Autodesk Inventor part; units mm, degrees
ref_plane "YZ Plane" through (0, 0, 0) normal (1, 0, 0) x (0, 1, 0)
ref_plane "XZ Plane" through (0, 0, 0) normal (0, 1, 0) x (-1, 0, 0)
ref_plane "XY Plane" through (0, 0, 0) normal (0, 0, 1) x (1, 0, 0)
sketch "Szkic2" plane through (0, 0, 0) normal (1, 0, 0) x (0, 1, 0)
  line L0 (0, -2.9) -> (0, 2.9)
  line L1 (-1.5, -1.5) -> (-1.5, 1.5)
  line L2 (-1.5, -1.5) -> (0, -2.9)
  line L3 (-1.5, 1.5) -> (0, 2.9)
  line L4 (0, 0) -> (-6, 0)
  line L5 (-6, 0) -> (-6, -1.5)
  line L6 (-6, -1.5) -> (-1.5, -1.5)
  dimension "d0" = 5.8
  dimension "d2" = 3
  dimension "d3" = 1.5
  dimension "d4" = 6
  dimension "d5" = 1.5
revolve "Obrót1" add sketch "Szkic2" angle 360 about axis through (0, 0, 0) along (0, -1, 0) contours L2 L1 L4 L0 | L6 L5 L4 L1
sketch "Szkic3" plane through (0, 0, 0) normal (0, 1, 0) x (1, 0, 0)
  line L0 (-1.1673, -0.633) -> (-1.1318, 0.6945)
  line L1 (-1.1318, 0.6945) -> (0.0355, 1.3274)
  line L2 (0.0355, 1.3274) -> (1.1673, 0.633)
  line L3 (1.1673, 0.633) -> (1.1318, -0.6945)
  line L4 (1.1318, -0.6945) -> (-0.0355, -1.3274)
  line L5 (-0.0355, -1.3274) -> (-1.1673, -0.633)
  point P0 (0, 0)
  point P1 (0, 0)
  dimension "d7" = 2.3
extrude "Wyciągnięcie proste1" cut sketch "Szkic3" against normal blind 2
fillet "Zaokrąglenie1" radius 0.5 6 edges at (-1.1496, -2, -0.0308) (-0.6014, -2, 0.9802) (-0.5482, -2, -1.011) (0.6014, -2, -0.9802) (0.5482, -2, 1.011) (1.1496, -2, 0.0308)
fillet "Zaokrąglenie2" radius 0.5 1 edges at (0, -1.5, 1.5)
fillet "Zaokrąglenie3" radius 0.1 1 edges at (0, 0, 2.9)
thread "Gwint1"
chamfer "Faza1" distance 0.5 angle 45 1 edges at (0, -6, 1.5)
properties part number "Screw M3 6mm flat head"
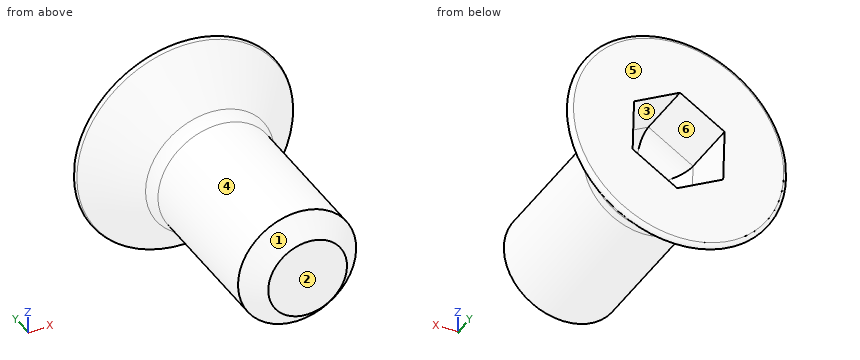
The listing builds one solid part. Answer for the finished solid, in the listing's coordinates (mm). Face numbers are marked on the shaded views. A direction names the side the tool comes from. Round coordinates to 2 decimals unless told otherwise and drop trailing zeros. Loops run counter-clockwise (first coordinate to the right, second up) from the corner with the lowest first, then second, coordinate; pieces in that order, holes last.
Q1. For a pull along X with two mould halves and no side action, classify the marked faces 1, 2 and 3 as released by +X, released by -X, zero draft, split by the parting line, or undercut.
Q2. Find the intervals of material crossed by line 1 (Y direction, x = 0.5, z = -0.25); line 2 (Z direction, x = -0.1, y = -0.5); line 3 (Z direction, x = -1.8, y = -0.6), in increasing order.
Q3. Given pin 1 Ø1.5 at (x, y) = (-0.5, -2.5) entering from +Z; pin 2 Ø1.5 at (y, z) = (-2, 2) entering from -X; pin 3 Ø3 at (x, y) = (2, -3.5) entering from -Z, each flat-ended and moving along its own axis, determine where each tip first touches the part or whether it passes through.
Q4. Which of the six approach directions +Z, -Z, +X, -X, +Y, -Y give full straight-line access (tool end or side, diameter ignored) to the marked faces 4, 5 and 6?
Q5. Section A-A, the plane y = -4.35 is taken. Determine the outline of the cut face in (x, z), then the cut area to 3 significant figures.
Completed:
1. face 1: split by the parting line
1. face 2: zero draft
1. face 3: undercut
2. line 1: y = -6 to -2
2. line 2: z = -2.43 to -1.25, 1.29 to 2.43
2. line 3: z = -1.5 to 1.5
3. pin 1: stops at z = 1.5
3. pin 2: stops at x = -0.83
3. pin 3: stops at z = -1.41
4. face 4: -Y
4. face 5: +Z, -Z, +X, -X, +Y
4. face 6: +Y
5. outline: circle Ø3 at (0, 0)
5. area: 7.07 mm2
